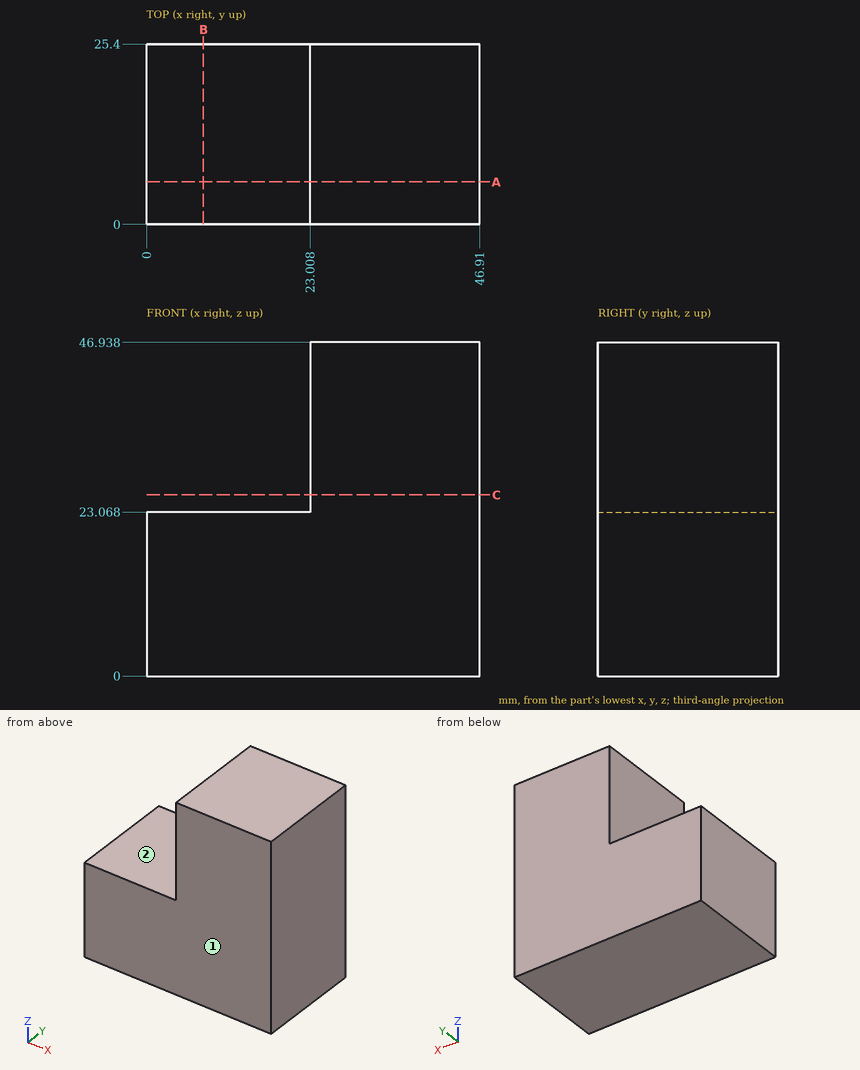
Geometry: see drawing. Coordinates: mm, zero at the bounding-box minimum. A direction names the side the tool comes from. Give positions to 0.01 mm unless a question says otherwise; leave off trailing zeros. Write each loop counter-clockwise with the first axis right and the second up, starting at its lowest first coordinate (ties: lowest second). Pieces come first, ordered by that corner, then holes. Notation, with made-up numbers: M 78.25,-7 L 83.25,-7 A18 cw 83.25,17 Z; hole C 77,17.5 d2. An arc over 180 degrees is marked long. Answer in a Markdown table with one row per item. Add a question column.
(1) Section C-C on z = 25.5. Return loops of the section in (x, y).
(2) Section B-B on x = 8. Return loops of the section in (y, z).
(3) Ray query, line 1 (Z direction, x = 2.5, y = 19.25); line 2 (X direction, y = 17, z = 26). Return the intervals inside material, ascending.
(4) Reachability of the marked faces 1 and 2 from +Z, -Z, +X, -X, +Y, -Y: full face, straight path, thin tool, end or side. Return the list, or none.
(5) First-contact query: pin 1 (6 mm diameter, centred on y = 14, z = 34.5, fed in from -X); pin 2 (11.5 mm diameter, centred on x = 12, y = 12.5, fed in from +Z). Flat tips, straight axial feed; report the tip coordinate or a pass-through.
(6) Section A-A on y = 6. Return loops of the section in (x, z).
Result set:
| question | item | result |
|---|---|---|
| 1 | outline | M 23.01,0 L 46.91,0 L 46.91,25.4 L 23.01,25.4 Z |
| 2 | outline | M 0,0 L 25.4,0 L 25.4,23.07 L 0,23.07 Z |
| 3 | line 1 | z = 0 to 23.07 |
| 3 | line 2 | x = 23.01 to 46.91 |
| 4 | face 1 | +Z, -Z, +X, -X, -Y |
| 4 | face 2 | +Z, -X, +Y, -Y |
| 5 | pin 1 | stops at x = 23.01 |
| 5 | pin 2 | stops at z = 23.07 |
| 6 | outline | M 0,0 L 46.91,0 L 46.91,46.94 L 23.01,46.94 L 23.01,23.07 L 0,23.07 Z |
